Here's how the part is built. I have some questions about the finished solid (model axes, mm). A direction names the side the tool comes from. Coordinates: 2 decimals unless noted, no trailing zeros. Loops run counter-clockwise (first coordinate to the right, second up) from the corner with the lowest first, then second, coordinate; pieces in that order, holes last.
```python
from build123d import *

# Parameters (mm, degrees)
SKETCH1_W           = 37
SKETCH1_H           = 37
SKETCH1_R           = 1.5
BOSS_EXTRUDE1_DEPTH = 3
SKETCH2_R           = 9
BOSS_EXTRUDE2_DEPTH = 2


with BuildPart() as part:
    # Sketch1 → Boss-Extrude1 (new body)
    with BuildSketch(Plane.XY):
        Rectangle(SKETCH1_W, SKETCH1_H)
        with Locations((15.5, 7.2)):
            Circle(SKETCH1_R, mode=Mode.SUBTRACT)
        with Locations((-15.5, 7.2)):
            Circle(SKETCH1_R, mode=Mode.SUBTRACT)
        with Locations((-15.5, 15.5)):
            Circle(SKETCH1_R, mode=Mode.SUBTRACT)
        with Locations((15.5, 15.5)):
            Circle(SKETCH1_R, mode=Mode.SUBTRACT)
        with Locations((15.5, -15.5)):
            Circle(SKETCH1_R, mode=Mode.SUBTRACT)
        with Locations((-15.5, -15.5)):
            Circle(SKETCH1_R, mode=Mode.SUBTRACT)
    extrude(amount=BOSS_EXTRUDE1_DEPTH)

    # Sketch2 → Boss-Extrude2 (add)
    with BuildSketch(Plane.XY.offset(3)):
        Circle(SKETCH2_R)
    extrude(amount=BOSS_EXTRUDE2_DEPTH)


solid = part.part
```
1. For pin 1 (2 mm diameter, centred on x = 6.5, y = 8.5, fed in from +Z); pin 2 (2.5 mm diameter, centred on x = -15.5, y = -15.5, fed in from -Z), each with a flat end and sliding along its axis, tell me the tip position at first contact or that it passes through.
2. On a 3-axis mill with a long thin cutter (end or side, diameter ignored), from which of +Z, -Z, +X, -X, +Y, -Y can I reach the whole of each face in a straight line? I mean faces 1 (the cylindrical face through (-1.172, 8.923, 3.986)), 2 (the cylindrical face through (-17, 15.57, 1.48)). Say none if no direction works.
3. I want a section at C-C (z = 1.85). Please give me the cut outline in (x, y), then the cut area to 3 significant figures.
4. We'd pull the mould along Y, two halves only. Please class faces 3 (the flat face through (0, 0, 0)), 4 (the cylindrical face through (14.3, 6.3, 1.5)), 5 (the flat face through (0, -18.5, 1)): +Y half, -Y half, draft (parallel to the pull), parting line (faces both ways), or undercut.
5. I want a section at B-B (x = -15.5). Please give me the cut outline in (y, z).
6. I need wall thicknesses on line 1 along Y through (x, z) = (15.5, 1.25); line 2 along Z through (x, y) = (15.5, 1.5); line 3 along X through (y, z) = (2, 3.7). Which ranges of each line are inside material? Lowest first, please.
7. I want a section at D-D (x = 0). Please give me the cut outline in (y, z), then the cut area to 3 significant figures.
8. I want a section at A-A (y = -15.5). Please give me the cut outline in (x, z).
Response values:
1. pin 1: stops at z = 3
1. pin 2: passes through
2. face 1: +Z
2. face 2: +Z, -Z
3. outline: (-18.5, -18.5) - (18.5, -18.5) - (18.5, 18.5) - (-18.5, 18.5) - close; hole circle Ø3 at (-15.5, -15.5); hole circle Ø3 at (-15.5, 7.2); hole circle Ø3 at (-15.5, 15.5); hole circle Ø3 at (15.5, -15.5); hole circle Ø3 at (15.5, 7.2); hole circle Ø3 at (15.5, 15.5)
3. area: 1,330 mm2
4. face 3: draft
4. face 4: undercut
4. face 5: -Y half
5. outline: (-18.5, 0) - (-17, 0) - (-17, 3) - (-18.5, 3) - close; (-14, 0) - (5.7, 0) - (5.7, 3) - (-14, 3) - close; (8.7, 0) - (14, 0) - (14, 3) - (8.7, 3) - close; (17, 0) - (18.5, 0) - (18.5, 3) - (17, 3) - close
6. line 1: y = -18.5 to -17, -14 to 5.7, 8.7 to 14, 17 to 18.5
6. line 2: z = 0 to 3
6. line 3: x = -8.77 to 8.77
7. outline: (-18.5, 0) - (18.5, 0) - (18.5, 3) - (9, 3) - (9, 5) - (-9, 5) - (-9, 3) - (-18.5, 3) - close
7. area: 147 mm2
8. outline: (-18.5, 0) - (-17, 0) - (-17, 3) - (-18.5, 3) - close; (-14, 0) - (14, 0) - (14, 3) - (-14, 3) - close; (17, 0) - (18.5, 0) - (18.5, 3) - (17, 3) - close
